Geometry: final body of the model. Coordinates: model frame, mm. Face numbers are marked on the shaded views. A direction names the side the tool comes from. Round coordinates to 2 decimals unless told otherwise and drop trailing zeros. Loops run counter-clockwise (first coordinate to the right, second up) from the corner with the lowest first, then second, coordinate; pieces in that order, holes last. Notation, with made-up numbers: M -25,-19.5 L 3,-19.5 A8 cw 3,-5.5 Z; hole C 79,6.5 d8. An arc over 180 degrees is marked long. Answer as a JSON object with one key per item and string values.
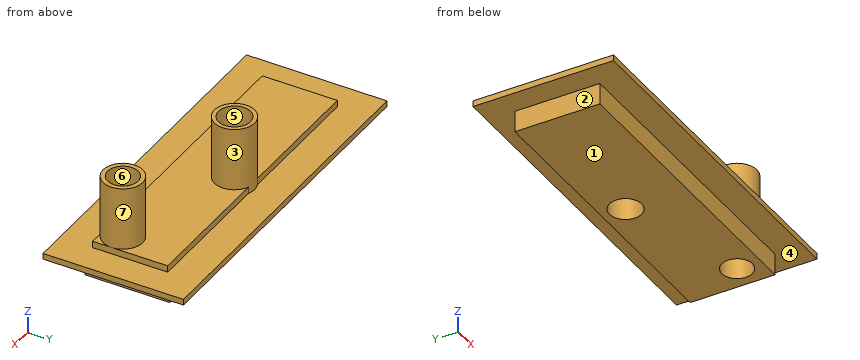
```python
from build123d import *

# Parameters (mm, degrees)
BOSS_EXTRUDE1_DEPTH     = 2.9718
BOSS_EXTRUDE2_DEPTH     = 3.302
BOSS_EXTRUDE3_DEPTH     = 10.668
SKETCH5_R               = 10.033
BOSS_EXTRUDE4_DEPTH     = 34.798
SKETCH4_R               = 9.8425
BOSS_EXTRUDE5_DEPTH     = 34.798
CUT_EXTRUDE1_DEPTH      = 107.07801353
CUT_EXTRUDE1_DEPTH_BACK = 107.07801353
SKETCH6_R               = 7.62
SKETCH6_R_2             = 8.001


with BuildPart() as part:
    # Sketch1 → Boss-Extrude1 (new body)
    with BuildSketch(Plane.XY):
        Polygon((-87.63, 35.03295), (87.63, 35.03295), (87.63, 0), (87.63, -35.03295), (0, -35.03295), (-87.63, -35.03295), (-87.63, 0), align=None)
    extrude(amount=BOSS_EXTRUDE1_DEPTH)

    # Sketch2 → Boss-Extrude2 (add)
    with BuildSketch(Plane.XY.offset(2.9718)):
        Polygon((-73.025, 18.7325), (73.025, 18.7325), (73.025, 0), (73.025, -18.7325), (0, -18.7325), (-73.025, -18.7325), (-73.025, 0), align=None)
    extrude(amount=BOSS_EXTRUDE2_DEPTH)

    # Sketch3 → Boss-Extrude3 (add)
    with BuildSketch(Plane(origin=(0, 0, 0), x_dir=(-1, 0, 0), z_dir=(0, 0, -1))):
        Polygon((-75.438, 21.209), (75.438, 21.209), (75.438, 0), (75.438, -21.209), (0, -21.209), (-75.438, -21.209), (-75.438, 0), align=None)
    extrude(amount=BOSS_EXTRUDE3_DEPTH)

    # Sketch5 → Boss-Extrude4 (add)
    with BuildSketch(Plane.XY.offset(2.9718)):
        with Locations(Location((-0.381, 9.50595, 0), (0, 0, 113.129371467))):
            Circle(SKETCH5_R)
    extrude(amount=BOSS_EXTRUDE4_DEPTH)

    # Sketch4 → Boss-Extrude5 (add)
    with BuildSketch(Plane.XY.offset(2.9718)):
        with Locations((63.1825, -9.31545)):
            Circle(SKETCH4_R)
    extrude(amount=BOSS_EXTRUDE5_DEPTH)

    # Sketch6 → Cut-Extrude1 (cut, two sides: drawn at the far end of the back side and taken through both)
    with BuildSketch(Plane.XY.offset(37.7698).offset(-CUT_EXTRUDE1_DEPTH_BACK)):
        with Locations((63.1825, -9.31545)):
            Circle(SKETCH6_R)
        with Locations((-0.381, 9.50595)):
            Circle(SKETCH6_R_2)
    extrude(amount=CUT_EXTRUDE1_DEPTH + CUT_EXTRUDE1_DEPTH_BACK, mode=Mode.SUBTRACT)


solid = part.part
```
1) Cut plane A-A on x = -43.5. Return the cut outline in (y, z).
Geometry results:
{"outline": "M -35.03,0 L -21.21,0 L -21.21,-10.67 L 21.21,-10.67 L 21.21,0 L 35.03,0 L 35.03,2.97 L 18.73,2.97 L 18.73,6.27 L -18.73,6.27 L -18.73,2.97 L -35.03,2.97 Z"}
2) Set-up query: the marked faces 1, 2 and 3. Return all of +Z, -Z, +X, -X, +Y, -Y with unobstructed straight access to the full face (end or side cutting, diameter ignored); none if empty.
Geometry results:
{"face 1": "-Z, +X, -X, +Y, -Y", "face 2": "-Z, -X, +Y, -Y", "face 3": "+Z"}
3) Pull-direction query (Y, two-part tool) for the marked faces 4, 5, 6 and 7; classes: +Y half, -Y half, draft (parallel to the pull), parting line (faces both ways), or undercut.
Geometry results:
{"face 4": "draft", "face 5": "undercut", "face 6": "undercut", "face 7": "parting line"}
4) Cut plane C-C on x = 64. Return the cut outline in (y, z).
Geometry results:
{"outline": "M -35.03,0 L -21.21,0 L -21.21,-10.67 L -16.89,-10.67 L -16.89,37.77 L -19.12,37.77 L -19.12,2.97 L -35.03,2.97 Z; M -1.74,-10.67 L 21.21,-10.67 L 21.21,0 L 35.03,0 L 35.03,2.97 L 18.73,2.97 L 18.73,6.27 L 0.49,6.27 L 0.49,37.77 L -1.74,37.77 Z"}
5) Line query: probe 1 along X at (y, z) = (-9, -4.5); probe 2 along Z at (x, y) = (12, 9); probe 3 along Y at (x, z) = (28, -7). Output: solid intervals per line, ascending.
Geometry results:
{"probe 1": "-75.44 to 55.57, 70.8 to 75.44", "probe 2": "-10.67 to 6.27", "probe 3": "-21.21 to 21.21"}
6) Cut plane D-D on z = 18. Return the cut outline in (x, y) (1 decimal), and give its area (3 significant figures).
Geometry results:
{"outline": "C -0.4,9.5 d20.1; C 63.2,-9.3 d19.7; hole C -0.4,9.5 d16; hole C 63.2,-9.3 d15.2", "area": "237 mm2"}
7) Cut plane B-B on y = 6. Return the cut outline in (x, z) (1 decimal), and give its area (3 significant figures).
Geometry results:
{"outline": "M -87.6,0 L -75.4,0 L -75.4,-10.7 L -7.6,-10.7 L -7.6,37.8 L -9.8,37.8 L -9.8,6.3 L -73,6.3 L -73,3 L -87.6,3 Z; M 6.8,-10.7 L 75.4,-10.7 L 75.4,0 L 87.6,0 L 87.6,3 L 73,3 L 73,6.3 L 9,6.3 L 9,37.8 L 6.8,37.8 Z", "area": "2,510 mm2"}
8) First-contact query: pin 1 (2.5 mm diameter, centred on y = 2, z = 5, fed in from -X) (3 decimals); pin 2 (3.5 mm diameter, centred on x = -35, z = 5, fed in from -Y); pin 3 (5.5 mm diameter, centred on x = -33, z = -8, fed in from +Y). Flat tips, straight axial feed; report the tip coordinate or a pass-through.
Geometry results:
{"pin 1": "x = -73.025", "pin 2": "y = -18.73", "pin 3": "y = 21.21"}
